from build123d import *

# Parameters (mm, degrees)
EXTRUDE_1_DEPTH = 10
M4X0_71_D       = 3.3
M3X0_51_D       = 2.5


with BuildPart() as part:
    # Эскиз1 → Бобышка-Вытянуть1 (new body)
    with BuildSketch(Plane(origin=(0, 0, 0), x_dir=(1, 0, 0), z_dir=(0, 1, 0))):
        with BuildLine():
            Line((0, 0), (41, 0))
            Line((41, 0), (41, 14.5))
            Line((41, 14.5), (32.959935794, 14.5))
            ThreePointArc((32.959935794, 14.5), (20.5, 3), (8.040064206, 14.5))
            Line((8.040064206, 14.5), (0, 14.5))
            Line((0, 14.5), (0, 0))
        make_face()
    extrude(amount=EXTRUDE_1_DEPTH)

    # Отверстие обработанное метчиком M4x0.71 (through all)
    with Locations(Plane(origin=(0, 0, -14.5), x_dir=(-1, 0, 0), z_dir=(0, 0, -1))):
        with Locations((-36.979967897, 5), (-4.020032103, 5)):
            Hole(M4X0_71_D / 2)

    # Отверстие обработанное метчиком M3x0.51 (through all)
    with Locations(Plane.XY):
        with Locations((20.5, 5)):
            Hole(M3X0_51_D / 2)


solid = part.part
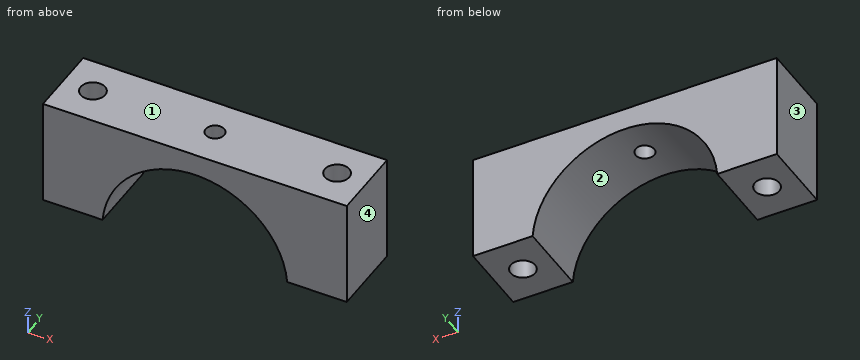
Source: CAD feature listing. Evaluate the final solid. Frame: model axes, mm. Face numbers are marked on the shaded views. Coordinates: 2 decimals unless noted, no trailing zeros. Order: outer loops, then holes, each group sorted by start corner. A loop starts at its lowest first (then second) coordinate and runs counter-clockwise, first axis right, second up. Notation, with made-up numbers: M 0.25,50 L 29.25,50 A26 cw 29.25,72 Z; hole C 53,76 d1. An arc over 180 degrees is marked long. Write each question's results on one line, items separated by ' | '. Start each with the question number.
Item 1: First-contact query: pin 1 Ø3 at (y, z) = (3.5, -3.5) entering from -X; pin 2 Ø5 at (x, y) = (19, 8.5) entering from -Z; pin 3 Ø3 at (x, y) = (36.98, 5) entering from +Z; pin 4 Ø1 at (x, y) = (25.5, 5) entering from -Z (3 decimals). Flat tips, straight axial feed; report the tip coordinate or a pass-through.
Item 2: Cut plane C-C (z = -1). Return loops of the section in (x, y), and give its area (3 significant figures).
Item 3: Line query: probe 1 along Y at (x, z) = (20.5, -1.1); probe 2 along X at (y, z) = (6, -10.75); probe 3 along X at (y, z) = (6.5, -8.5). Output: solid intervals per line, ascending.
Item 4: Cut plane B-B (z = -6.5). Return loops of the section in (x, y), and give its area (3 significant figures).
Item 5: Cut plane D-D (y = 5). Return loops of the section in (x, z).
Item 6: Cut plane A-A (x = 20.5). Return loops of the section in (y, z), and give its area (3 significant figures).
Item 7: Draft query along X for the marked faces 1, 2, 3 and 4. Return one class per face: pulls with the +X half, pulls with the -X half, needs draft (parallel to the pull), parting line crosses it, or undercut.
Checked values:
1) pin 1: stops at x = 0 | pin 2: stops at z = -3.66 | pin 3: passes through | pin 4: stops at z = -4.275
2) outline: M 0,0 L 41,0 L 41,10 L 0,10 Z; hole C 4.02,5 d3.3; hole C 20.5,5 d2.5; hole C 36.98,5 d3.3 | area: 388 mm2
3) probe 1: y = 0 to 3.75, 6.25 to 10 | probe 2: x = 0 to 2.71, 5.33 to 8.94, 32.06 to 35.67, 38.29 to 41 | probe 3: x = 0 to 3.33, 4.71 to 10.14, 30.86 to 36.29, 37.67 to 41
4) outline: M 0,0 L 11.83,0 L 11.83,10 L 0,10 Z; M 29.17,0 L 41,0 L 41,10 L 29.17,10 Z; hole C 4.02,5 d3.3; hole C 36.98,5 d3.3 | area: 219 mm2
5) outline: M 0,-14.5 L 2.37,-14.5 L 2.37,0 L 0,0 Z; M 5.67,-14.5 L 8.04,-14.5 A12.5 cw 19.25,-3.06 L 19.25,0 L 5.67,0 Z; M 21.75,-3.06 A12.5 cw 32.96,-14.5 L 35.33,-14.5 L 35.33,0 L 21.75,0 Z; M 38.63,-14.5 L 41,-14.5 L 41,0 L 38.63,0 Z
6) outline: M 0,-3 L 3.75,-3 L 3.75,0 L 0,0 Z; M 6.25,-3 L 10,-3 L 10,0 L 6.25,0 Z | area: 22.5 mm2
7) face 1: needs draft | face 2: undercut | face 3: pulls with the -X half | face 4: pulls with the +X half
